```python
from build123d import *

# Parameters (mm, degrees)
SKETCH1_R                = 0.75
BOSS_EXTRUDE1_DEPTH      = 10
BOSS_EXTRUDE2_DEPTH      = 1
BOSS_EXTRUDE2_DEPTH_BACK = 1
FILLET1_R                = 1
SKETCH3_R                = 0.6
CUT_EXTRUDE1_DEPTH       = 5


with BuildPart() as part:
    # Sketch1 → Boss-Extrude1 (new body)
    with BuildSketch(Plane(origin=(0, 0, 0), x_dir=(0, 0, -1), z_dir=(1, 0, 0))):
        Circle(SKETCH1_R)
    extrude(amount=BOSS_EXTRUDE1_DEPTH)

    # Sketch2 → Boss-Extrude2 (add, two sides: drawn at the far end of the back side and taken through both)
    with BuildSketch(Plane(origin=(0, 0, 0), x_dir=(1, 0, 0), z_dir=(0, 1, 0)).offset(-BOSS_EXTRUDE2_DEPTH_BACK)):
        Polygon((1, 1.875), (1, -1.875), (-3, -1.875), (-3, -0.875), (0, -0.875), (0, 0.875), (-3, 0.875), (-3, 1.875), align=None)
    extrude(amount=BOSS_EXTRUDE2_DEPTH + BOSS_EXTRUDE2_DEPTH_BACK)

    # Fillet1
    fillet1_edges = [part.edges().sort_by_distance(p)[0] for p in [
        (-3, 1, -1.375),
        (-3, -1, -1.375),
        (-3, -1, 1.375),
        (-3, 1, 1.375),
        (1, 0, -1.875),
        (1, 0, 1.875),
    ]]
    fillet(fillet1_edges, radius=FILLET1_R - 0.0001)  # a hair under: the kernel refuses the full size

    # Sketch3 → Cut-Extrude1 (cut)
    with BuildSketch(Plane(origin=(0, 0, -1.875), x_dir=(-1, 0, 0), z_dir=(0, 0, -1))):
        with Locations((1.7, 0)):
            Circle(SKETCH3_R)
    extrude(amount=-CUT_EXTRUDE1_DEPTH, mode=Mode.SUBTRACT)


solid = part.part
```
Can you work these out from the model? Positions are in its coordinate system, mm. A direction names the side the tool comes from. Give positions to 0.01 mm unless a question says otherwise; leave off trailing zeros. Write each loop counter-clockwise with the first axis right and the second up, starting at its lowest first coordinate (ties: lowest second). Pieces come first, ordered by that corner, then holes. Notation, with made-up numbers: (-6.5, 24) - (0.5, 24) arc R16 ccw to (0.5, 33) - close; hole circle Ø4 at (17, -35.75). An arc over 180 degrees is marked (long way). Write item = value, one per line. Start each with the question number.
1. Imagine slicing it at C-C (y = 0.2). Please give me the cut outline in (x, z) (3 decimals), and give its area (3 significant figures).
2. Thinking about a two-plate mould opening in Y: for faces 4 (the face through (-1.1, 0, -1.4)), 5 (the face through (0, 0, 0)), 6 (the face through (0.2, -1, 0)), which applies, released by +Y, released by -Y, zero draft, split by the parting line, or undercut?
3. Imagine slicing it at A-A (x = -1.7). Please give me the cut outline in (y, z) (3 decimals).
4. Imagine slicing it at B-B (z = 0.6). Please give me the cut outline in (x, y).
5. On a 3-axis mill with a long thin cutter (end or side, diameter ignored), from which of +Z, -Z, +X, -X, +Y, -Y can I reach the whole of each face in a straight line? I mean faces 1 (the face through (5.44, 0.03, 0.75)), 2 (the face through (-1.1, 0, 1.4)), 3 (the face through (-0.9, 0, 0.875)). Say none if no direction works.
6. Please list where these lines run through material, in increasing order: line 1 (Z direction, x = -1, y = -0.5) (3 decimals); line 2 (Y direction, x = -1.7, z = 1.55); line 3 (X direction, y = -0.4, z = 0.45).
Worked answers:
q1.outline = (-2.98, -1.875) - (-2.266, -1.875) - (-2.266, -0.875) - (-2.98, -0.875) - close; (-2.98, 0.875) - (-2.266, 0.875) - (-2.266, 1.875) - (-2.98, 1.875) - close; (-1.134, -1.875) - (0, -1.875) arc R1 ccw to (1, -0.875) - (1, -0.723) - (10, -0.723) - (10, 0.723) - (1, 0.723) - (1, 0.875) arc R1 ccw to (0, 1.875) - (-1.134, 1.875) - (-1.134, 0.875) - (0, 0.875) - (0, -0.875) - (-1.134, -0.875) - close
q1.area = 20.0 mm2
q2.face_4 = undercut
q2.face_5 = zero draft
q2.face_6 = released by -Y
q3.outline = (-1, -1.875) - (-0.6, -1.875) - (-0.6, -0.875) - (-1, -0.875) - close; (-1, 0.875) - (-0.6, 0.875) - (-0.6, 1.875) - (-1, 1.875) - close; (0.6, -1.875) - (1, -1.875) - (1, -0.875) - (0.6, -0.875) - close; (0.6, 0.875) - (1, 0.875) - (1, 1.875) - (0.6, 1.875) - close
q4.outline = (0, -1) - (1, -1) - (1, -0.45) - (10, -0.45) - (10, 0.45) - (1, 0.45) - (1, 1) - (0, 1) - close
q5.face_1 = +X
q5.face_2 = +Z, -Z
q5.face_3 = -X, +Y, -Y
q6.line_1 = -1.875 to -0.875, 0.875 to 1.875
q6.line_2 = -1 to -0.6, 0.6 to 1
q6.line_3 = 0 to 10
